Could you check a few things on this model? Use its own coordinates, in mm. A direction names the side the tool comes from. Coordinates: 2 decimals unless noted, no trailing zeros. Loops run counter-clockwise (first coordinate to the right, second up) from the corner with the lowest first, then second, coordinate; pieces in that order, holes last.
from build123d import *

# Parameters (mm, degrees)
SKETCH2_W           = 38
SKETCH2_H           = 19.1
SKETCH2_R           = 6.55
SKETCH2_R_2         = 2
BOSS_EXTRUDE1_DEPTH = 2.5
SKETCH3_R           = 2
SKETCH3_W           = 13.5
SKETCH3_H           = 13.1
BOSS_EXTRUDE2_DEPTH = 6
BOSS_EXTRUDE3_DEPTH = 5
SKETCH5_W           = 2
SKETCH5_H           = 4
BOSS_EXTRUDE4_DEPTH = 13.5


with BuildPart() as part:
    # Sketch2 → Boss-Extrude1 (new body)
    with BuildSketch(Plane.XY):
        Rectangle(SKETCH2_W, SKETCH2_H)
        with Locations((9.45, 0)):
            Circle(SKETCH2_R, mode=Mode.SUBTRACT)
        Circle(SKETCH2_R_2, mode=Mode.SUBTRACT)
    extrude(amount=-BOSS_EXTRUDE1_DEPTH)

    # Sketch3 → Boss-Extrude2 (add)
    with BuildSketch(Plane(origin=(0, 0, -2.5), x_dir=(-1, 0, 0), z_dir=(0, 0, -1))):
        Polygon((-19, -9.55), (19, -9.55), (19, -5.55), (2.5, -5.55), (2.5, 5.55), (19, 5.55), (19, 9.55), (-19, 9.55), align=None)
        with Locations(Location((0, 0, 0), (0, 0, 180))):
            Circle(SKETCH3_R, mode=Mode.SUBTRACT)
        with Locations((-9.25, 0)):
            Rectangle(SKETCH3_W, SKETCH3_H, mode=Mode.SUBTRACT)
    extrude(amount=BOSS_EXTRUDE2_DEPTH)

    # Sketch4 → Boss-Extrude3 (add)
    with BuildSketch(Plane(origin=(0, 0, -8.5), x_dir=(-1, 0, 0), z_dir=(0, 0, -1))):
        Polygon((19, 5.55), (16.5, 5.55), (16.5, 7.05), (-16.5, 7.05), (-16.5, -7.05), (16.5, -7.05), (16.5, -5.55), (19, -5.55), (19, -9.55), (-19, -9.55), (-19, 9.55), (19, 9.55), align=None)
    extrude(amount=BOSS_EXTRUDE3_DEPTH)

    # Sketch5 → Boss-Extrude4 (add)
    with BuildSketch(Plane(origin=(0, 0, -13.5), x_dir=(-1, 0, 0), z_dir=(0, 0, -1))):
        with Locations((-20, 7.55)):
            Rectangle(SKETCH5_W, SKETCH5_H)
        with Locations((-20, -7.55)):
            Rectangle(SKETCH5_W, SKETCH5_H)
    boss_extrude4 = extrude(amount=-BOSS_EXTRUDE4_DEPTH)

    # Mirror1: Boss-Extrude4 across plane
    add(boss_extrude4.mirror(Plane(origin=(0, 0, 0), x_dir=(0, 0, 1), z_dir=(1, 0, 0))))


solid = part.part
(1) Imagine slicing it at A-A, the plane z = -8. Write out the boundary of the cut face in (x, y).
Answers:
outline: (-21, -9.55) - (21, -9.55) - (21, -5.55) - (19, -5.55) - (19, 5.55) - (21, 5.55) - (21, 9.55) - (-21, 9.55) - (-21, 5.55) - (-2.5, 5.55) - (-2.5, -5.55) - (-21, -5.55) - close; hole circle Ø4 at (0, 0); hole (2.5, -6.55) - (16, -6.55) - (16, 6.55) - (2.5, 6.55) - close
(2) We'd pull the mould along Y, two halves only. Please class faces 1 (the face through (2.5, 0, -5)), 2 (the face through (-5, 0, 0)), 3 (the face through (0, -9.55, -7)): +Y half, -Y half, draft (parallel to the pull), parting line (faces both ways), or undercut.
Answers:
face 1: undercut
face 2: draft
face 3: -Y half
(3) Imagine slicing it at D-D, the plane x = -14. Write out the boundary of the cut face in (y, z), and give its area (3 significant figures).
Answers:
outline: (-9.55, -13.5) - (-7.05, -13.5) - (-7.05, -8.5) - (-5.55, -8.5) - (-5.55, -2.5) - (5.55, -2.5) - (5.55, -8.5) - (7.05, -8.5) - (7.05, -13.5) - (9.55, -13.5) - (9.55, 0) - (-9.55, 0) - close
area: 121 mm2
(4) Imagine slicing it at C-C, the plane y = -0.5. State how many separate pieces and enclosed holes the cut face has, and give its area (3 significant figures).
Answers:
separate pieces: 3
enclosed holes: 0
area: 89.9 mm2
(5) Imagine slicing it at B-B, the plane x = 0. Write out the boundary of the cut face in (y, z), and give its area (3 significant figures).
Answers:
outline: (-9.55, -13.5) - (-7.05, -13.5) - (-7.05, -8.5) - (-2, -8.5) - (-2, 0) - (-9.55, 0) - close; (2, -8.5) - (7.05, -8.5) - (7.05, -13.5) - (9.55, -13.5) - (9.55, 0) - (2, 0) - close
area: 153 mm2
(6) Which directions (+Z, -Z, +X, -X, +Y, -Y) give clear straight access to the entire face, cutting with the end or side of a thin tool? Please do faces 4 (the face through (19, 0, -7)), 5 (the face through (-14, -5.55, -7)), 6 (the face through (2.906, 0.288, -1.232)), 7 (the face through (-21, 8, -7)), 8 (the face through (-16.5, -6, -11)).
Answers:
face 4: +Z, -Z, +X
face 5: -Z, -X
face 6: +Z, -Z
face 7: +Z, -Z, -X, +Y, -Y
face 8: -Z
(7) I need wall thicknesses on probe 1 along X at (y, z) = (-5.25, -7.25); probe 2 along Y at (x, z) = (0, -5.6); probe 3 along Y at (x, z) = (-18, -9.75). Which ranges of each line are inside material? Lowest first, please.
Answers:
probe 1: x = -2.5 to 2.5, 16 to 19
probe 2: y = -9.55 to -2, 2 to 9.55
probe 3: y = -9.55 to -5.55, 5.55 to 9.55
(8) For pin 1 (3 mm diameter, centred on y = -0.5, z = -1.5, fed in from -X); pin 2 (2.5 mm diameter, centred on y = -0.5, z = -11.5, fed in from -X); pin 3 (3 mm diameter, centred on x = -7, y = 4, fed in from -Z), each with a flat end and sliding along its axis, tell me the tip position at first contact or that it passes through.
Answers:
pin 1: stops at x = -19
pin 2: stops at x = 16.5
pin 3: stops at z = -2.5
